Geometry check sheet. Reference: the model listing, model coordinates, mm. Coordinates: 2 decimals unless noted, no trailing zeros. Order: outer loops, then holes, each group sorted by start corner. A loop starts at its lowest first (then second) coordinate and runs counter-clockwise, first axis right, second up.
```python
from build123d import *

# Parameters (mm, degrees)
SKETCH1_W           = 90
SKETCH1_H           = 90
SKETCH1_R           = 4.1656
BOSS_EXTRUDE1_DEPTH = 3
SKETCH2_R           = 9.144
CUT_EXTRUDE1_DEPTH  = 7
CUT_EXTRUDE1_TAPER  = 45


with BuildPart() as part:
    # Sketch1 → Boss-Extrude1 (new body, symmetric)
    with BuildSketch(Plane.XY):
        with Locations((45, 45)):
            Rectangle(SKETCH1_W, SKETCH1_H)
        with Locations((22.5, 45)):
            Circle(SKETCH1_R, mode=Mode.SUBTRACT)
        with Locations((67.5, 45)):
            Circle(SKETCH1_R, mode=Mode.SUBTRACT)
    extrude(amount=BOSS_EXTRUDE1_DEPTH, both=True)

    # Sketch2 → Cut-Extrude1 (cut, through all)
    with BuildSketch(Plane.XY.offset(3)):
        with Locations((22.5, 45)):
            Circle(SKETCH2_R)
        with Locations((67.5, 45)):
            Circle(SKETCH2_R)
    extrude(amount=-CUT_EXTRUDE1_DEPTH, taper=CUT_EXTRUDE1_TAPER, mode=Mode.SUBTRACT)


solid = part.part
```
Item 1: Thickness scan on line 1 along X through (y, z) = (45, -2.7); line 2 along Y through (x, z) = (67.5, -2.2); line 3 along X through (y, z) = (48.5, -2.5). Record the ranges inside material, lowest first.
Item 2: Release check for a two-part mould opening along X. For faces 1 (the face through (44, 0, 0)), 2 (the face through (21.54, 40.7, -1.74)), 3 (the face through (0, 44, 0)) record: pulls with the +X half, pulls with the -X half, needs draft (parallel to the pull), parting line crosses it, or undercut.
Item 3: Sectioned sample at B-B (y = 45). Give the number of separate pieces and of enclosed holes in the cut face, and give its area (3 significant figures).
Item 4: Sectioned sample at A-A (x = 22.5). Record the cut outline in (y, z), and give its area (3 significant figures).
Item 5: Depth check by flat-ended pin: P1, Ø11, axis at x = 67.5, y = 45, coming from the +Z side; P2, Ø13.5, axis at x = 22.5, y = 45, coming from the +Z side. Enter the tip coordinate at first touch or a pass-through.
Item 6: Sectioned sample at C-C (z = -0.25). Record the cut outline in (x, y).
Geometry check:
1. line 1: x = 0 to 18.33, 26.67 to 63.33, 71.67 to 90
1. line 2: y = 0 to 40.83, 49.17 to 90
1. line 3: x = 0 to 20.24, 24.76 to 65.24, 69.76 to 90
2. face 1: needs draft
2. face 2: undercut
2. face 3: pulls with the -X half
3. separate pieces: 3
3. enclosed holes: 0
3. area: 390 mm2
4. outline: (0, -3) - (40.83, -3) - (40.83, -1.98) - (35.86, 3) - (0, 3) - close; (49.17, -3) - (90, -3) - (90, 3) - (54.14, 3) - (49.17, -1.98) - close
4. area: 465 mm2
5. P1: stops at z = -0.64
5. P2: stops at z = 0.61
6. outline: (0, 0) - (90, 0) - (90, 90) - (0, 90) - close; hole circle Ø11.79 at (22.5, 45); hole circle Ø11.79 at (67.5, 45)
